Could you check a few things on this drawing? It's one solid part, dimensions in mm from its lowest x, y, z. Coordinates: 2 decimals unless noted, no trailing zeros. Write each loop counter-clockwise with the first axis right and the second up, starting at its lowest first coordinate (ties: lowest second). Pieces come first, ordered by that corner, then holes. Notation, with made-up numbers: (-21, 58) - (-11, 58) arc R9 ccw to (-11, 74) - close; hole circle Ø11 at (46, 22). An arc over 180 degrees is marked (long way). Answer as a JSON object with one key per item and string values. Group by question number.
1) If we section it at B-B (y = 0.65): Write out the boundary of the cut face in (x, z).
2) If we section it at A-A (x = 72): Write out the boundary of the cut face in (y, z).
3) Will these pins go through, and if not, where does the flat tip stop? pin 1 Ø1 at (y, z) = (1, 32.5) entering from +X; pin 2 Ø0.8 at (x, y) = (1.5, 0.5) entering from +Z; pin 3 Ø0.8 at (y, z) = (1.5, 140) entering from -X.
4) Please list where these lines run through material, in increasing order: line 1 along Z through (x, y) = (76.5, 0.65); line 2 along X through (y, z) = (1.35, 20); line 3 along Z through (x, y) = (118.5, 1.05).
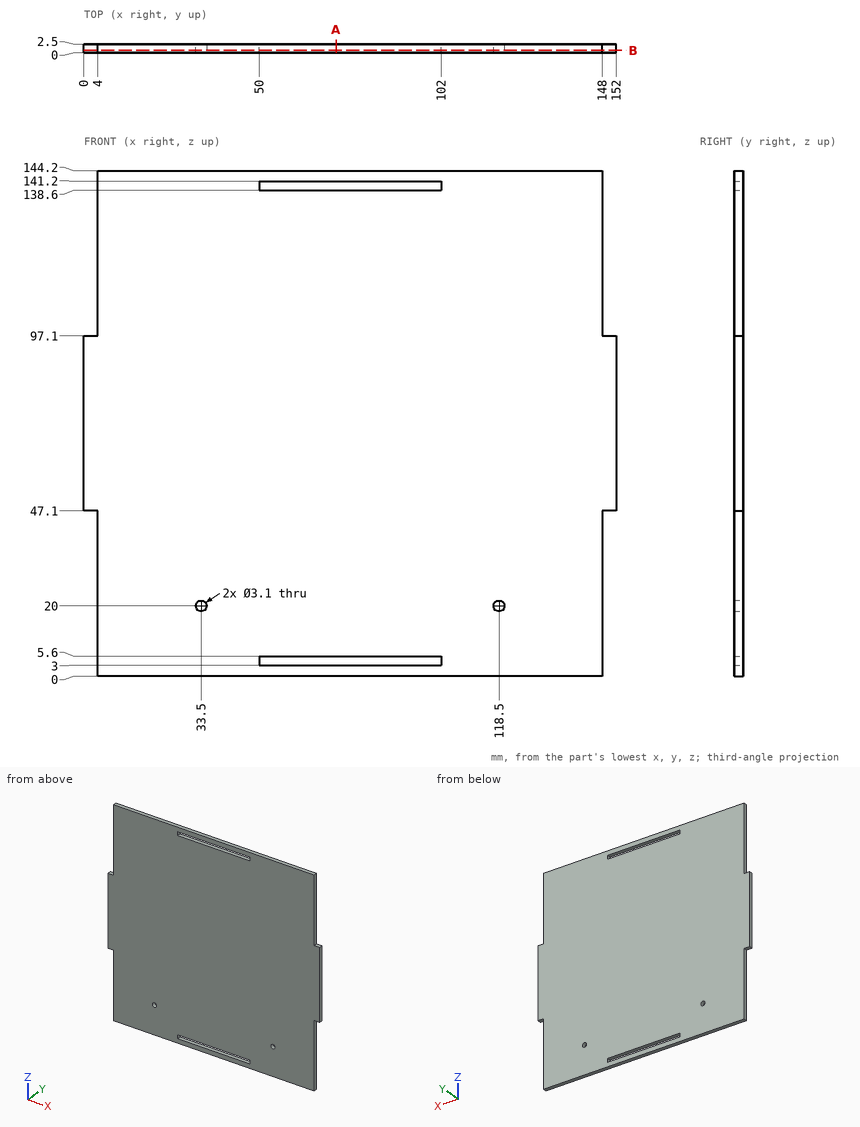
Here are the results:
{
 "1": {"outline": "(0, 47.1) - (4, 47.1) - (4, 0) - (148, 0) - (148, 47.1) - (152, 47.1) - (152, 97.1) - (148, 97.1) - (148, 144.2) - (4, 144.2) - (4, 97.1) - (0, 97.1) - close; hole circle Ø3.1 at (33.5, 20); hole (50, 3) - (102, 3) - (102, 5.6) - (50, 5.6) - close; hole (50, 138.6) - (102, 138.6) - (102, 141.2) - (50, 141.2) - close; hole circle Ø3.1 at (118.5, 20)"},
 "2": {"outline": "(0, 0) - (2.5, 0) - (2.5, 3) - (0, 3) - close; (0, 5.6) - (2.5, 5.6) - (2.5, 138.6) - (0, 138.6) - close; (0, 141.2) - (2.5, 141.2) - (2.5, 144.2) - (0, 144.2) - close"},
 "3": {"pin 1": "stops at x = 148", "pin 2": "stops at z = 97.1", "pin 3": "stops at x = 4"},
 "4": {"line 1": "z = 0 to 3, 5.6 to 138.6, 141.2 to 144.2", "line 2": "x = 4 to 31.95, 35.05 to 116.95, 120.05 to 148", "line 3": "z = 0 to 18.45, 21.55 to 144.2"}
}
